Geometry check sheet. Reference: the model listing, model coordinates, mm. Coordinates: 2 decimals unless noted, no trailing zeros. Order: outer loops, then holes, each group sorted by start corner. A loop starts at its lowest first (then second) coordinate and runs counter-clockwise, first axis right, second up. Notation, with made-up numbers: (74, 87.5) - (94, 87.5) arc R23 cw to (94, 123.5) - close; hole circle Ø10 at (-1.75, 39). An arc over 180 degrees is marked (long way). Return JSON: item names as keys, results as strings. Group by question number.
Item 1: Scan lines: probe 1 along Z at (x, y) = (0.85, 8.5); probe 2 along Z at (x, y) = (3.6, 26.5); probe 3 along Y at (x, z) = (3.55, 30.5). Record each from-to range of solid material in increasing order.
Item 2: Section check A-A on y = 14. Enter the section's corners in (x, z).
Item 3: Gauge pin test, flat ends, axial feed: pin 1 (6.5 mm diameter, centred on y = -20, z = 45, fed in from -X); pin 2 (1.2 mm diameter, centred on x = 0.5, y = 19.5, fed in from -Z); pin 3 (1.5 mm diameter, centred on x = 0.5, y = 4, fed in from +Z). Record the tip position at first contact, or that the pin passes through.
Item 4: Section check D-D on z = 45. Give the number of separate pieces and of enclosed holes in the cut face, then the cut area to 3 significant figures.
Item 5: Section check C-C on x = 1.2. Enter the section's corners in (y, z).
Item 6: Section check B-B on z = -17. Enter the section's corners in (x, y).
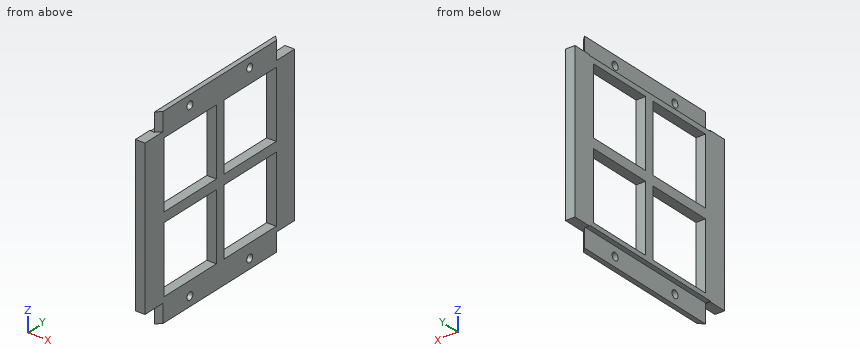
Autodesk Inventor part; units mm, degrees
ref_plane "YZ Plane" through (0, 0, 0) normal (1, 0, 0) x (0, 1, 0)
ref_plane "XZ Plane" through (0, 0, 0) normal (0, 1, 0) x (-1, 0, 0)
ref_plane "XY Plane" through (0, 0, 0) normal (0, 0, 1) x (1, 0, 0)
sketch "Sketch1" plane through (0, 0, 0) normal (1, 0, 0) x (0, 1, 0)
  line L0 (-40.43, 50) -> (40.43, 50)
  line L1 (50, 40.43) -> (50, -40.43)
  line L2 (40.43, -50) -> (-40.43, -50)
  line L3 (-50, -40.43) -> (-50, 40.43)
  line L4 (40.43, 50) -> (40.43, 40.43)
  line L5 (40.43, 40.43) -> (50, 40.43)
  line L6 (-50, 40.43) -> (-40.43, 40.43)
  line L7 (-40.43, 40.43) -> (-40.43, 50)
  line L8 (-40.43, -50) -> (-40.43, -40.43)
  line L9 (-40.43, -40.43) -> (-50, -40.43)
  line L10 (50, -40.43) -> (40.43, -40.43)
  line L11 (40.43, -40.43) -> (40.43, -50)
  line L12 (2.75, 2.3115) -> (37.75, 2.3115)
  line L13 (37.75, 2.3115) -> (37.75, 37.3115)
  line L14 (37.75, 37.3115) -> (2.75, 37.3115)
  line L15 (2.75, 37.3115) -> (2.75, 2.3115)
  line L16 (2.75, -37.6885) -> (37.75, -37.6885)
  line L17 (2.75, -2.6885) -> (2.75, -37.6885)
  line L18 (37.75, -2.6885) -> (2.75, -2.6885)
  line L19 (37.75, -37.6885) -> (37.75, -2.6885)
  line L20 (-37.25, 2.3115) -> (-2.25, 2.3115)
  line L21 (-37.25, 37.3115) -> (-37.25, 2.3115)
  line L22 (-2.25, 37.3115) -> (-37.25, 37.3115)
  line L23 (-2.25, 2.3115) -> (-2.25, 37.3115)
  line L24 (-37.25, -37.6885) -> (-2.25, -37.6885)
  line L25 (-37.25, -2.6885) -> (-37.25, -37.6885)
  line L26 (-2.25, -2.6885) -> (-37.25, -2.6885)
  line L27 (-2.25, -37.6885) -> (-2.25, -2.6885)
  line L28 (40.43, 40.43) -> (50, 40.43)
  line L29 (50, 40.43) -> (50, 50)
  line L30 (50, 50) -> (40.43, 50)
  line L31 (40.43, 50) -> (40.43, 40.43)
  line L32 (40.43, -40.43) -> (50, -40.43)
  line L33 (50, -40.43) -> (50, -50)
  line L34 (50, -50) -> (40.43, -50)
  line L35 (40.43, -50) -> (40.43, -40.43)
  line L36 (-40.43, -40.43) -> (-50, -40.43)
  line L37 (-50, -40.43) -> (-50, -50)
  line L38 (-50, -50) -> (-40.43, -50)
  line L39 (-40.43, -50) -> (-40.43, -40.43)
  line L40 (-40.43, 40.43) -> (-50, 40.43)
  line L41 (-50, 40.43) -> (-50, 50)
  line L42 (-50, 50) -> (-40.43, 50)
  line L43 (-40.43, 50) -> (-40.43, 40.43)
  circle A0 centre (20.0008, 45) radius 2
  circle A1 centre (20.0008, -45) radius 2
  circle A2 centre (-19.9992, 45) radius 2
  circle A3 centre (-19.9992, -45) radius 2
  point P0 (0, 0)
  point P1 (50, 45.215)
  dimension "d7" = 9.57
  dimension "d8" = 9.57
  dimension "d11" = 360
  dimension "d13" = 80.86
  dimension "d14" = 100
  dimension "d15" = 35
  dimension "d16" = 35
  dimension "d19" = 40
  dimension "d22" = 40
  dimension "d25" = 4
  dimension "d26" = 30
  dimension "d27" = 5
  dimension "d30" = 90
  dimension "d33" = 40
  dimension "d36" = 12.25
extrude "Extrusion1" add sketch "Sketch1" along normal blind 5 contours L0 L4 L5 L1 L10 L11 L2 L8 L9 L3 L6 L7
sketch "Sketch2" plane through (0, -40.43, 50) normal (0, 0, 1) x (1, 0, 0)
  line L0 (0, -9.57) -> (0, 0)
  line L1 (0, 80.86) -> (5, 80.86)
  line L2 (0, 0) -> (2.5, 0)
  line L3 (2.5, 0) -> (2.5, 80.86)
  line L4 (2.5, 80.86) -> (0, 80.86)
  line L5 (0, 80.86) -> (0, 0)
  point P0 (0, 40.43)
extrude "Extrusion2" cut sketch "Sketch2" against normal blind 10
sketch "Sketch3" plane through (0, -40.43, -50) normal (0, 0, -1) x (-1, 0, 0)
  line L0 (-2.5, 80.86) -> (-2.5, 0)
  line L1 (0, 0) -> (-2.5, 0)
  line L2 (-2.5, 0) -> (-2.5, 80.86)
  line L3 (-2.5, 80.86) -> (0, 80.86)
  line L4 (0, 80.86) -> (0, 0)
  point P0 (0, 40.43)
extrude "Extrusion3" cut sketch "Sketch3" against normal blind 10
chamfer "Chamfer3" distance 2.5 angle 45 4 edges at (5, -40.43, 45.215) (5, 40.43, 45.215) (5, -40.43, -45.215) (5, 40.43, -45.215)
properties part number "Side Panel"
Computed:
{
 "1": {"probe 1": "z = -40 to -37.69, -2.69 to 2.31, 37.31 to 40", "probe 2": "z = -50 to -37.69, -2.69 to 2.31, 37.31 to 50", "probe 3": "y = -50 to -37.25, -2.25 to 2.75, 37.75 to 50"},
 "2": {"outline": "(0, -40) - (2.5, -40) - (2.5, -50) - (5, -50) - (5, -37.69) - (0, -37.69) - close; (0, -2.69) - (5, -2.69) - (5, 2.31) - (0, 2.31) - close; (0, 37.31) - (5, 37.31) - (5, 50) - (2.5, 50) - (2.5, 40) - (0, 40) - close"},
 "3": {"pin 1": "stops at x = 2.5", "pin 2": "stops at z = -40", "pin 3": "stops at z = 40"},
 "4": {"separate pieces": "3", "enclosed holes": "0", "area": "176 mm²"},
 "5": {"outline": "(-50, -40.43) - (-40.43, -40.43) - (-40.43, -40) - (40.43, -40) - (40.43, -40.43) - (50, -40.43) - (50, 40.43) - (40.43, 40.43) - (40.43, 40) - (-40.43, 40) - (-40.43, 40.43) - (-50, 40.43) - close; hole (-37.25, -37.69) - (-2.25, -37.69) - (-2.25, -2.69) - (-37.25, -2.69) - close; hole (-37.25, 2.31) - (-2.25, 2.31) - (-2.25, 37.31) - (-37.25, 37.31) - close; hole (2.75, -37.69) - (37.75, -37.69) - (37.75, -2.69) - (2.75, -2.69) - close; hole (2.75, 2.31) - (37.75, 2.31) - (37.75, 37.31) - (2.75, 37.31) - close"},
 "6": {"outline": "(0, -50) - (5, -50) - (5, -37.25) - (0, -37.25) - close; (0, -2.25) - (5, -2.25) - (5, 2.75) - (0, 2.75) - close; (0, 37.75) - (5, 37.75) - (5, 50) - (0, 50) - close"}
}
